from build123d import *

# Parameters (mm, degrees)
SKETCH1_R           = 1.25
SKETCH1_R_2         = 1.75
BOSS_EXTRUDE2_DEPTH = 5


with BuildPart() as part:
    # Sketch1 → Boss-Extrude2 (new body)
    with BuildSketch(Plane.XY):
        with BuildLine():
            Line((349.257683179, 374.699911371), (348.046522548, 372.418831878))
            Line((348.046522548, 372.418831878), (346.468308818, 374.536137019))
            Line((346.468308818, 374.536137019), (345.55259362, 372.121245841))
            Line((345.55259362, 372.121245841), (343.721455877, 374.024052769))
            Line((343.721455877, 374.024052769), (343.115627486, 371.513434183))
            Line((343.115627486, 371.513434183), (341.060443866, 373.171734495))
            Line((341.060443866, 373.171734495), (340.774056559, 370.604982455))
            Line((340.774056559, 370.604982455), (338.527238535, 371.992623765))
            Line((338.527238535, 371.992623765), (338.564808811, 369.410217484))
            Line((338.564808811, 369.410217484), (336.161790046, 370.505315861))
            Line((336.161790046, 370.505315861), (336.522725398, 367.947981428))
            Line((336.522725398, 367.947981428), (334.001402933, 368.733266515))
            Line((334.001402933, 368.733266515), (334.680011196, 366.241334623))
            Line((334.680011196, 366.241334623), (332.080147792, 366.704422005))
            Line((332.080147792, 366.704422005), (333.065726908, 364.317191908))
            Line((333.065726908, 364.317191908), (330.428323965, 364.450778421))
            Line((330.428323965, 364.450778421), (331.705330762, 362.205898164))
            Line((331.705330762, 362.205898164), (329.0719817, 362.007877067))
            Line((329.0719817, 362.007877067), (330.620277019, 359.940749753))
            Line((330.620277019, 359.940749753), (328.032511325, 359.414243959))
            Line((328.032511325, 359.414243959), (329.827677623, 357.55746942))
            Line((329.827677623, 357.55746942), (327.326305908, 356.71078224))
            Line((327.326305908, 356.71078224), (329.34003234, 355.093642919))
            Line((329.34003234, 355.093642919), (326.964502731, 353.940127114))
            Line((326.964502731, 353.940127114), (329.165031629, 352.588126266))
            Line((329.165031629, 352.588126266), (326.952807646, 351.145973471))
            Line((326.952807646, 351.145973471), (329.305435355, 350.080432955))
            Line((329.305435355, 350.080432955), (327.291405091, 348.37238678))
            Line((327.291405091, 348.37238678), (329.759029266, 347.610110808))
            Line((329.759029266, 347.610110808), (327.974955183, 345.663108161))
            Line((327.974955183, 345.663108161), (330.518659917, 345.21611828))
            Line((330.518659917, 345.21611828), (328.992677928, 343.060864557))
            Line((328.992677928, 343.060864557), (331.572347478, 342.936210064))
            Line((331.572347478, 342.936210064), (330.328523231, 340.606694904))
            Line((330.328523231, 340.606694904), (332.903474666, 340.806341675))
            Line((332.903474666, 340.806341675), (331.961424013, 338.339302922))
            Line((331.961424013, 338.339302922), (334.491048812, 338.860102409))
            Line((334.491048812, 338.860102409), (333.865628454, 336.294446739))
            Line((333.865628454, 336.294446739), (336.310032922, 337.128185622))
            Line((336.310032922, 337.128185622), (336.011106111, 334.504374958))
            Line((336.011106111, 334.504374958), (338.331740529, 335.637904676))
            Line((338.331740529, 335.637904676), (338.364021521, 332.997318079))
            Line((338.364021521, 332.997318079), (340.524288099, 334.412762192))
            Line((340.524288099, 334.412762192), (340.887267801, 331.797043291))
            Line((340.887267801, 331.797043291), (342.853097845, 333.4720794))
            Line((342.853097845, 333.4720794), (343.541051852, 330.922479643))
            Line((343.541051852, 330.922479643), (344.568787794, 332.049317014))
            Line((344.568787794, 332.049317014), (346.321351139, 292.508956491))
            ThreePointArc((346.321351139, 292.508956491), (351.821351139, 287.008956491), (357.321351139, 292.508956491))
            Line((357.321351139, 292.508956491), (357.299783306, 292.995557967))
            Line((357.299783306, 292.995557967), (355.520486612, 333.139061449))
            Line((355.520486612, 333.139061449), (357.268666905, 331.728478036))
            Line((357.268666905, 331.728478036), (357.555054212, 334.295230076))
            Line((357.555054212, 334.295230076), (359.801872235, 332.907588766))
            Line((359.801872235, 332.907588766), (359.76430196, 335.489995047))
            Line((359.76430196, 335.489995047), (362.167320725, 334.394896671))
            Line((362.167320725, 334.394896671), (361.806385373, 336.952231103))
            Line((361.806385373, 336.952231103), (364.327707838, 336.166946016))
            Line((364.327707838, 336.166946016), (363.649099575, 338.658877908))
            Line((363.649099575, 338.658877908), (366.248962979, 338.195790526))
            Line((366.248962979, 338.195790526), (365.263383863, 340.583020623))
            Line((365.263383863, 340.583020623), (367.900786806, 340.449434111))
            Line((367.900786806, 340.449434111), (366.623780008, 342.694314367))
            Line((366.623780008, 342.694314367), (369.257129071, 342.892335464))
            Line((369.257129071, 342.892335464), (367.708833752, 344.959462778))
            Line((367.708833752, 344.959462778), (370.296599446, 345.485968572))
            Line((370.296599446, 345.485968572), (368.501433148, 347.342743111))
            Line((368.501433148, 347.342743111), (371.002804863, 348.189430292))
            Line((371.002804863, 348.189430292), (368.98907843, 349.806569612))
            Line((368.98907843, 349.806569612), (371.36460804, 350.960085417))
            Line((371.36460804, 350.960085417), (369.164079142, 352.312086265))
            Line((369.164079142, 352.312086265), (371.376303125, 353.754239061))
            Line((371.376303125, 353.754239061), (369.023675416, 354.819779576))
            Line((369.023675416, 354.819779576), (371.03770568, 356.527825751))
            Line((371.03770568, 356.527825751), (368.570081505, 357.290101724))
            Line((368.570081505, 357.290101724), (370.354155588, 359.23710437))
            Line((370.354155588, 359.23710437), (367.810450854, 359.684094251))
            Line((367.810450854, 359.684094251), (369.336432842, 361.839347974))
            Line((369.336432842, 361.839347974), (366.756763293, 361.964002467))
            Line((366.756763293, 361.964002467), (368.00058754, 364.293517627))
            Line((368.00058754, 364.293517627), (365.425636104, 364.093870857))
            Line((365.425636104, 364.093870857), (366.367686758, 366.560909609))
            Line((366.367686758, 366.560909609), (363.838061959, 366.040110123))
            Line((363.838061959, 366.040110123), (364.463482317, 368.605765792))
            Line((364.463482317, 368.605765792), (362.019077849, 367.77202691))
            Line((362.019077849, 367.77202691), (362.31800466, 370.395837574))
            Line((362.31800466, 370.395837574), (359.997370241, 369.262307855))
            Line((359.997370241, 369.262307855), (359.96508925, 371.902894452))
            Line((359.96508925, 371.902894452), (357.804822672, 370.487450339))
            Line((357.804822672, 370.487450339), (357.441842969, 373.103169241))
            Line((357.441842969, 373.103169241), (355.476012926, 371.428133131))
            Line((355.476012926, 371.428133131), (354.788058919, 373.977732888))
            Line((354.788058919, 373.977732888), (353.047667725, 372.069521103))
            Line((353.047667725, 372.069521103), (352.045588858, 374.512793004))
            Line((352.045588858, 374.512793004), (350.558083522, 372.401499183))
            Line((350.558083522, 372.401499183), (349.257683179, 374.699911371))
        make_face()
        with Locations((351.821351139, 292.508956491)):
            Circle(SKETCH1_R, mode=Mode.SUBTRACT)
        with Locations((349.164555385, 352.450106266)):
            Circle(SKETCH1_R_2, mode=Mode.SUBTRACT)
    extrude(amount=BOSS_EXTRUDE2_DEPTH)


solid = part.part
For this review, take the finished solid that the model builds, in its own axes (mm). Give positions to 0.01 mm unless a question says otherwise; leave off trailing zeros. Order: outer loops, then holes, each group sorted by start corner. A loop starts at its lowest first (then second) coordinate and runs counter-clockwise, first axis right, second up. Notation, with made-up numbers: (-36, 70.5) - (1, 70.5) arc R15 cw to (1, 90.5) - close; hole circle Ø11 at (37.25, -21.75). An arc over 180 degrees is marked (long way). Answer as a JSON object with one key per item and string values. Group by question number.
Item 1: Clearance check with flat-ended pins moving along their axes: pin 1 Ø1.5 at (x, y) = (351.82, 292.51) entering from -Z; pin 2 Ø1.5 at (y, z) = (319.5, 2) entering from +X; pin 3 Ø2 at (x, z) = (343, 1.5) entering from +Y; pin 4 Ø3 at (x, z) = (361.5, 3) entering from -Y. State where each tip first meets the part, or that it passes through.
Item 2: Take a section at A-A on z = 4.25. Give the number of separate pieces and of enclosed holes in the cut face, and give its area (3 significant figures).
Item 3: Wall thickness on line 1 along Y through (x, z) = (333, 0.9); line 2 along Y through (x, z) = (351.5, 2.25); line 3 along X through (y, z) = (330.5, 3): over which ranges is each line inside the solid? List them lowest first.
Item 4: Draft analysis for pull direction X (two halves, no side actions). For faces 1 (the flat face through (352.554, 373.274, 2.465)), 2 (the flat face through (340.92, 371.91, 2.46)), state which applies: pulls with the +X half, pulls with the -X half, needs draft (parallel to the pull), parting line crosses it, or undercut.
Item 5: Take a section at C-C on y = 304. Give the boundary of the cut face in (x, z).
Item 6: Take a section at B-B on x = 354. Give the boundary of the cut face in (y, z), and give its area (3 significant figures).
Reported:
{
 "1": {"pin 1": "through", "pin 2": "x = 356.16", "pin 3": "y = 374.02", "pin 4": "y = 334.39"},
 "2": {"separate pieces": "1", "enclosed holes": "2", "area": "1,860 mm^2"},
 "3": {"line 1": "338.55 to 364.32, 364.48 to 366.54", "line 2": "287.02 to 291.3, 293.72 to 373.74", "line 3": "344.64 to 355.64"},
 "4": {"face 1": "undercut", "face 2": "undercut"},
 "5": {"outline": "(345.81, 0) - (356.81, 0) - (356.81, 5) - (345.81, 5) - close"},
 "6": {"outline": "(287.46, 0) - (373.11, 0) - (373.11, 5) - (287.46, 5) - close", "area": "428 mm^2"}
}
